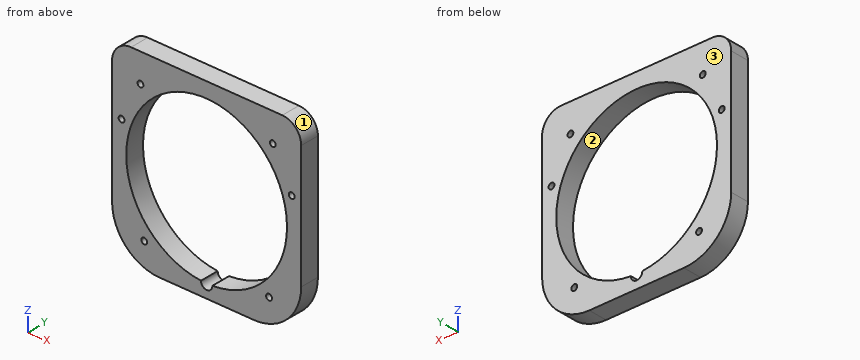
```python
from build123d import *

# Parameters (mm, degrees)
DODANIE_WYCI_GNI_CIE1_DEPTH = 10
WYTNIJ_WYCI_GNI_CIE2_DEPTH  = 142.774468788
SZKIC5_R                    = 1.55
WYTNIJ_WYCI_GNI_CIE3_DEPTH  = 142.774468788


with BuildPart() as part:
    # Szkic1 → Dodanie-wyciągnięcie1 (new body)
    with BuildSketch(Plane(origin=(0, 0, 0), x_dir=(1, 0, 0), z_dir=(0, 1, 0))):
        with BuildLine():
            Line((10, 0), (90, 0))
            ThreePointArc((90, 0), (97.071067812, 2.928932188), (100, 10))
            Line((100, 10), (100, 75))
            ThreePointArc((100, 75), (92.67766953, 92.67766953), (75, 100))
            Line((75, 100), (25, 100))
            ThreePointArc((25, 100), (7.32233047, 92.67766953), (0, 75))
            Line((0, 75), (0, 10))
            ThreePointArc((0, 10), (2.928932188, 2.928932188), (10, 0))
        make_face()
    extrude(amount=-DODANIE_WYCI_GNI_CIE1_DEPTH)

    # Szkic4 → Wytnij-wyciągnięcie2 (cut, through all)
    with BuildSketch(Plane(origin=(0, 0, 0), x_dir=(1, 0, 0), z_dir=(0, 1, 0))):
        with BuildLine():
            ThreePointArc((47.001869094, 92.855975693), (50, 7.961858046), (52.998130906, 92.855975693))
            ThreePointArc((52.998130906, 92.855975693), (50, 95.961858046), (47.001869094, 92.855975693))
        make_face()
    extrude(amount=-WYTNIJ_WYCI_GNI_CIE2_DEPTH, mode=Mode.SUBTRACT)

    # Szkic5 → Wytnij-wyciągnięcie3 (cut, through all)
    with BuildSketch(Plane(origin=(0, 0, 0), x_dir=(1, 0, 0), z_dir=(0, 1, 0))):
        with Locations(Location((83, 86.378345537, 0), (0, 0, 270))):
            Circle(SZKIC5_R)
        with Locations(Location((85, 15, 0), (0, 0, 270))):
            Circle(SZKIC5_R)
        with Locations(Location((5, 35, 0), (0, 0, 270))):
            Circle(SZKIC5_R)
        with Locations(Location((95, 35, 0), (0, 0, 270))):
            Circle(SZKIC5_R)
        with Locations(Location((17, 86.378345537, 0), (0, 0, 270))):
            Circle(SZKIC5_R)
        with Locations(Location((15, 15, 0), (0, 0, 270))):
            Circle(SZKIC5_R)
    extrude(amount=-WYTNIJ_WYCI_GNI_CIE3_DEPTH, mode=Mode.SUBTRACT)


solid = part.part
```
Source: CAD feature listing. Evaluate the final solid. Frame: model axes, mm. Face numbers are marked on the shaded views. Give positions to 0.01 mm unless a question says otherwise; leave off trailing zeros. Write each loop counter-clockwise with the first axis right and the second up, starting at its lowest first coordinate (ties: lowest second). Pieces come first, ordered by that corner, then holes. Notation, with made-up numbers: (69, 47) - (119, 47) arc R20 ccw to (119, 77) - close; hole circle Ø2 at (21.5, -28.75). An arc over 180 degrees is marked (long way). One line per item, written item: value. Start each with the question number.
Q1. Section query C-C, the plane y = -4.25. Return the cut outline in (x, z), then the cut area to 3 significant figures.
Q2. Section query A-A, the plane x = 50. Return the cut outline in (y, z).
Q3. Section query B-B, the plane z = -40.5. Return the cut outline in (x, y), then the cut area to 3 significant figures.
Q4. Material intervals for probe 1 along X at (y, z) = (-2.75, -35); probe 2 along X at (y, z) = (-2, -15); probe 3 along Z at (x, y) = (50.5, -1.25), sorted ascending. Write a range as from..to.
Q5. Draft query along Z for the marked faces 1, 2 and 3. Return one class per face: +Z half, -Z half, draft (parallel to the pull), parting line (faces both ways), or undercut.
Q6. First-contact query: pin 1 Ø2 at (x, z) = (20.5, -23) entering from +Y. Flat tip, straight axial feed; report the tip coordinate or a pass-through.
Answer:
1. outline: (0, -75) arc R25 ccw to (25, -100) - (75, -100) arc R25 ccw to (100, -75) - (100, -10) arc R10 ccw to (90, 0) - (10, 0) arc R10 ccw to (0, -10) - close; hole circle Ø3.1 at (5, -35); hole circle Ø3.1 at (15, -15); hole circle Ø3.1 at (17, -86.38); hole (47, -92.86) arc R3 ccw (long way) to (53, -92.86) arc R42.5 ccw (long way) to start; hole circle Ø3.1 at (83, -86.38); hole circle Ø3.1 at (85, -15); hole circle Ø3.1 at (95, -35)
1. area: 3,950 mm2
2. outline: (-10, -100) - (0, -100) - (0, -95.96) - (-10, -95.96) - close; (-10, -7.96) - (0, -7.96) - (0, 0) - (-10, 0) - close
3. outline: (0, -10) - (8.68, -10) - (8.68, 0) - (0, 0) - close; (91.32, -10) - (100, -10) - (100, 0) - (91.32, 0) - close
3. area: 174 mm2
4. probe 1: x = 0..3.45, 6.55..10.41, 89.59..93.45, 96.55..100
4. probe 2: x = 0..13.45, 16.55..26.58, 73.42..83.45, 86.55..100
4. probe 3: z = -100..-95.92, -7.96..0
5. face 1: +Z half
5. face 2: undercut
5. face 3: draft
6. pin 1: passes through
